Build history of the part. All positions in model axes, mm. A direction names the side the tool comes from. Give positions to 0.01 mm unless a question says otherwise; leave off trailing zeros.
1) 3-axis set-ups, long thin cutter, end or side, ignore diameter. For faces 1 (the cylindrical face through (5, -1.36, -30.82)), 2 (the flat face through (0, 27, 17)), 3 (the cylindrical face through (3.796, -11.339, 36.007)), 4 (the flat face through (10.5, 24, -20)): which of +Z, -Z, +X, -X, +Y, -Y reach the whole face in a straight line?
2) Flat gauge pins, fed straight in: P1, Ø6, axis at x = 6.5, y = 1, coming from the -Z side; P2, Ø1, axis at x = 4.5, z = 26.5, coming from the -Y side; P3, Ø2, axis at x = 8.5, y = 12, coming from the -Z side. Where does each tip first touch, or does it go through?
3) Two-plate mould, pull along Y, no slides. Class faces 5 (the flat face through (11.5, -34, -14)), 6 (the conical face through (9.237, 29.247, -6.495)), 7 (the cylindrical face through (0.85, -1.36, -30.82)), 8 (the conical face through (7.219, -11.358, 36.066)): +Y half, -Y half, draft (parallel to the pull), parting line (faces both ways), or undercut.
4) Wall check: line 1 (Y direction, x = 1, z = 0); line 2 (Y direction, x = 9, z = 2.5); line 3 (Y direction, x = 8, z = -18). Give the ranges that are in metal, low to high.
```python
from build123d import *

# Parameters (mm, degrees)
FILLET1_R = 0.5


with BuildPart() as part:
    # Sketch1 → Revolve1 (revolve)
    with BuildSketch(Plane.XY, mode=Mode.PRIVATE) as revolve1_sk:
        with BuildLine():
            Line((0, 30.85), (0, 37.75))
            Line((0, 37.75), (7, 37.75))
            Line((7, 37.75), (10.5, 38.75))
            Line((10.5, 38.75), (11.5, 37.75))
            Line((11.5, 37.75), (11.5, 36.25))
            Line((11.5, 36.25), (8.224507889, 35.311303332))
            ThreePointArc((8.224507889, 35.311303332), (7.500003732, 34.347267981), (8.229764579, 33.387205724))
            Line((8.229764579, 33.387205724), (10.5, 32.75))
            Line((10.5, 32.75), (10.5, 31))
            Line((10.5, 31), (9.4, 29.9))
            Line((9.4, 29.9), (6.8, 30.85))
            Line((6.8, 30.85), (3.25, 30.85))
            Line((3.25, 30.85), (2.5, 30.1))
            Line((2.5, 30.1), (1.200961894, 30.85))
            Line((1.200961894, 30.85), (0, 30.85))
        make_face()
    revolve(revolve1_sk.sketch.rotate(Axis((0, 0, 0), (1, 0, 0)), 90), axis=Axis((0, 0, 0), (1, 0, 0)))

    # Fillet1
    fillet1_edges = [part.edges().sort_by_distance(p)[0] for p in [
        (0, 0, -30.85),
        (0, 0, -37.75),
    ]]
    fillet(fillet1_edges, radius=FILLET1_R)


solid = part.part
```
Findings below:
1. face 1: none
1. face 2: +Z, -Z, -X, +Y, -Y
1. face 3: -X
1. face 4: +X
2. P1: stops at z = -38.45
2. P2: stops at y = -27.37
2. P3: stops at z = -36.68
3. face 5: draft
3. face 6: undercut
3. face 7: undercut
3. face 8: parting line
4. line 1: y = -37.75 to -30.85, 30.85 to 37.75
4. line 2: y = -38.24 to -35.45, -33.08 to -29.94, 29.94 to 33.08, 35.45 to 38.24
4. line 3: y = -33.51 to -30.27, -28.23 to -24.51, 24.51 to 28.23, 30.27 to 33.51
